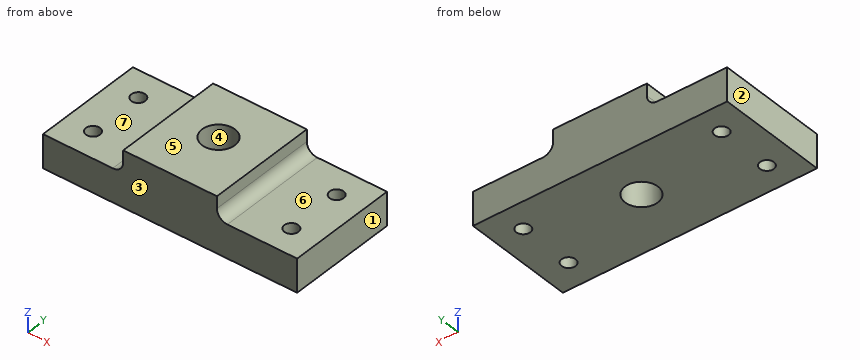
```python
from build123d import *

# Parameters (mm, degrees)
F0_W      = 144.4625
F0_H      = 31.6992
F1_DEPTH  = 62.992
F2_W      = 45.60062
F2_H      = 12.7762
F3_DEPTH  = 62.993
F4_R      = 5.95376
F5_R      = 9.3091
F6_DEPTH  = 31.7002
F7_R      = 3.96875
F7_R_2    = 3.9751
F8_DEPTH  = 18.924
F9_R      = 3.96875
F10_DEPTH = 18.924


with BuildPart() as f1:
    # F0 (on Front) → F1 (new body)
    with BuildSketch(Plane.XZ):
        Rectangle(F0_W, F0_H)
    extrude(amount=F1_DEPTH)

    # F2 (on face) → F3 (cut, through all)
    with BuildSketch(Plane.XZ.offset(62.992)):
        with Locations((-49.43094, 9.4615)):
            Rectangle(F2_W, F2_H)
        with Locations((49.43094, 9.4615)):
            Rectangle(F2_W, F2_H)
    extrude(amount=-F3_DEPTH, mode=Mode.SUBTRACT)

    # F4
    f4_edges = [f1.edges().sort_by_distance(p)[0] for p in [
        (-26.63063, -31.496, 3.0734),
        (26.63063, -31.496, 3.0734),
    ]]
    fillet(f4_edges, radius=F4_R)

    # F5 (on face) → F6 (cut, through all)
    with BuildSketch(Plane.XY.offset(15.8496)):
        with Locations((0, -29.0322)):
            Circle(F5_R)
    extrude(amount=-F6_DEPTH, mode=Mode.SUBTRACT)

    # F7 (on face) → F8 (cut, through all)
    with BuildSketch(Plane.XY.offset(3.0734)):
        with Locations((-56.38165, -15.7226)):
            Circle(F7_R)
        with Locations((-56.38165, -47.4726)):
            Circle(F7_R_2)
    extrude(amount=-F8_DEPTH, mode=Mode.SUBTRACT)

    # F9 (on face) → F10 (cut, through all)
    with BuildSketch(Plane.XY.offset(3.0734)):
        with Locations((56.38165, -15.7226)):
            Circle(F9_R)
        with Locations((56.38165, -47.4726)):
            Circle(F9_R)
    extrude(amount=-F10_DEPTH, mode=Mode.SUBTRACT)


solid = f1.part
```
Read the model definition and answer for the solid it produces. Units are mm, in the model's axes. Face numbers are marked on the shaded views. A direction names the side the tool comes from. Coordinates: 2 decimals unless noted, no trailing zeros. Order: outer loops, then holes, each group sorted by start corner. A loop starts at its lowest first (then second) coordinate and runs counter-clockwise, first axis right, second up. Notation, with made-up numbers: (25, 82.25) - (46, 82.25) arc R12 cw to (46, 100.25) - close; hole circle Ø3 at (86.5, 71). An arc over 180 degrees is marked (long way). Answer as a JSON object with one key per item and string values. Group by question number.
Item 1: Section D-D (z = 7) is taken. Give the vertices of the cut face in (x, y).
Item 2: Consider probe 1 along X at (y, z) = (-18, -5); probe 2 along Y at (x, z) = (0, -9); probe 3 along Z at (x, y) = (-62, -45.5). Determine where each line is inside the solid, lowest interval first. Write a range as from..to.
Item 3: Section A-A (x = 0) is taken. Give the vertices of the cut face in (y, z).
Item 4: A tool of negligible diameter and unlimited length cuts with its end or side. For the marked faces 5, 6 and 7, from which of +Z, -Z, +X, -X, +Y, -Y can it reach the whole face along a straight path? Write none if from no direction.
Item 5: Section C-C (y = -30.5) is taken. Give the vertices of the cut face in (x, z).
Item 6: Flat-ended cylindrical pins translate along their axes: P1, Ø12, axis at x = -34.5, y = -36, coming from the +Z side; P2, Ø6, axis at y = -23, z = 7.5, coming from the -X side; P3, Ø5, axis at x = 56.38, y = -15.72, coming from the +Z side; P4, Ø6, axis at y = -50.5, z = 7.5, coming from the +X side. Find the tip coordinate at first contact, or state that the pin passes through.
Item 7: The mould has two halves that part along X. Classify the marked faces 1, 2, 3 and 4: +X half, -X half, draft (parallel to the pull), parting line (faces both ways), or undercut.
Item 8: Section B-B (z = -5) is taken. Give the vertices of the cut face in (x, y), plus the area to 3 significant figures.
Results are:
{
 "1": {"outline": "(-26.99, -62.99) - (26.99, -62.99) - (26.99, 0) - (-26.99, 0) - close; hole circle Ø18.62 at (0, -29.03)"},
 "2": {"probe 1": "x = -72.23..-59.63, -53.13..53.13, 59.63..72.23", "probe 2": "y = -62.99..-38.34, -19.72..0", "probe 3": "z = -15.85..3.07"},
 "3": {"outline": "(-62.99, -15.85) - (-38.34, -15.85) - (-38.34, 15.85) - (-62.99, 15.85) - close; (-19.72, -15.85) - (0, -15.85) - (0, 15.85) - (-19.72, 15.85) - close"},
 "4": {"face 5": "+Z, +X, -X, +Y, -Y", "face 6": "+Z, +X, +Y, -Y", "face 7": "+Z, -X, +Y, -Y"},
 "5": {"outline": "(-72.23, -15.85) - (-9.19, -15.85) - (-9.19, 15.85) - (-26.63, 15.85) - (-26.63, 9.03) arc R5.95 cw to (-32.58, 3.07) - (-72.23, 3.07) - close; (9.19, -15.85) - (72.23, -15.85) - (72.23, 3.07) - (32.58, 3.07) arc R5.95 cw to (26.63, 9.03) - (26.63, 15.85) - (9.19, 15.85) - close"},
 "6": {"P1": "stops at z = 4.7", "P2": "stops at x = -28.72", "P3": "passes through", "P4": "stops at x = 28.72"},
 "7": {"face 1": "+X half", "face 2": "-X half", "face 3": "draft", "face 4": "undercut"},
 "8": {"outline": "(-72.23, -62.99) - (72.23, -62.99) - (72.23, 0) - (-72.23, 0) - close; hole circle Ø7.95 at (-56.38, -47.47); hole circle Ø7.94 at (-56.38, -15.72); hole circle Ø18.62 at (0, -29.03); hole circle Ø7.94 at (56.38, -47.47); hole circle Ø7.94 at (56.38, -15.72)", "area": "8,630 mm^2"}
}
